Verification items for this drawing (mm, ordinates from the low corner). A direction names the side the tool comes from. Coordinates: 2 decimals unless noted, no trailing zeros. Order: outer loops, then holes, each group sorted by start corner. A loop starts at its lowest first (then second) coordinate and runs counter-clockwise, first axis right, second up. Notation, with made-up numbers: (23.25, 71.5) -> (31.25, 71.5) arc R27 ccw to (31.25, 98.5) -> close; hole circle Ø11 at (-31, 14). An arc over 180 degrees is marked (long way). Write each question's results on one line, items separated by ' | '. Start each with the question number.
(1) Cross-section at D-D on y = 17.75. Enter the section's corners in (x, z).
(2) Cross-section at C-C on y = 2. Enter the section's corners in (x, z) (1 decimal), and give its area (3 significant figures).
(3) Set-up check for the marked faces 1, 2, 3, 4 and 5: record each of +Z, -Z, +X, -X, +Y, -Y from which the full face is reachable in a straight line by a thin tool's end or side.
(4) Thickness scan on probe 1 along Y at (x, z) = (11, 11); probe 2 along X at (y, z) = (1, 9) (3 decimals); probe 3 along Z at (x, y) = (4.5, 2.25). Record the ranges inside material, lowest first. Write a range as [from, to].
(5) Cross-section at A-A on z = 7.5. Enter the section's corners in (x, y) (3 decimals).
(6) Go/stop test with flat-tipped pins: pin 1 (4 mm diameter, centred on y = 10, z = 8, fed in from -X); pin 2 (6 mm diameter, centred on y = 9.5, z = 1.5, fed in from +X) (1 decimal); pin 3 (1.1 mm diameter, centred on y = 2, z = 8, fed in from -X) (3 decimals). Record where each tip stops, or that it passes through.
(7) Cross-section at B-B on x = 9. Enter the section's corners in (y, z).
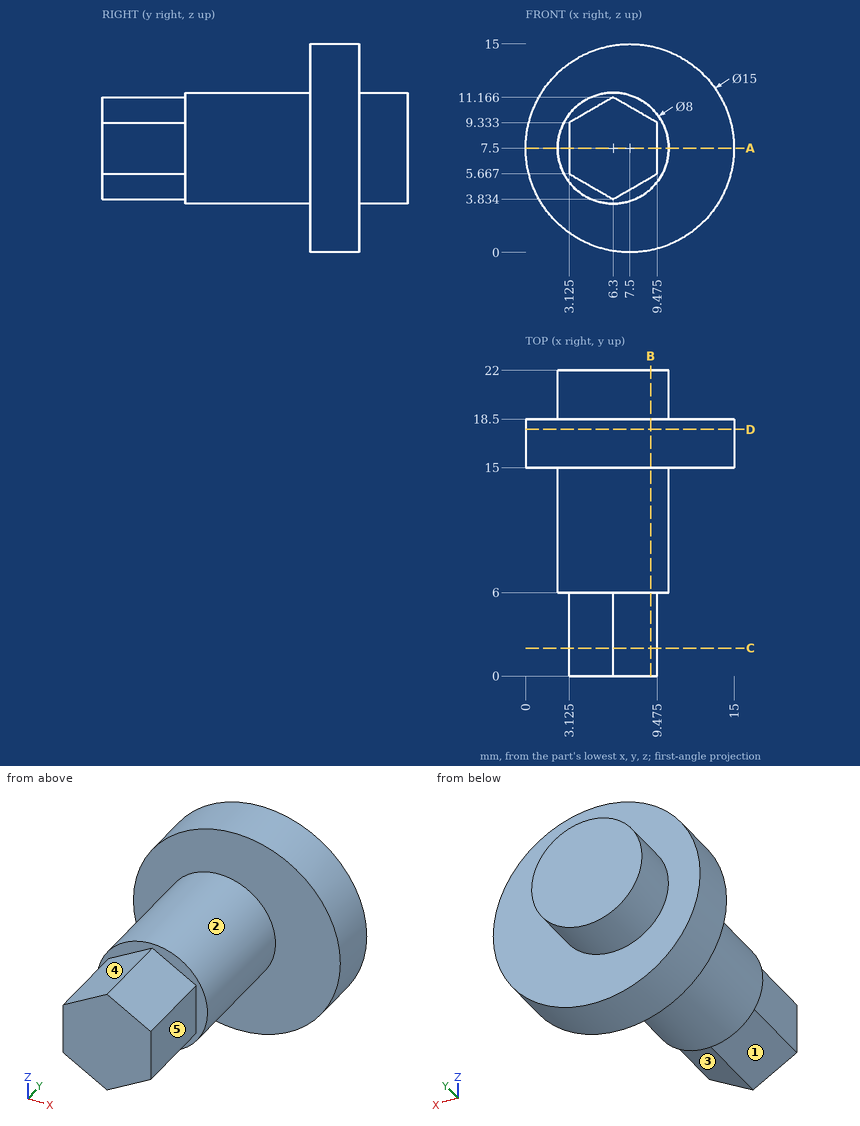
Results are:
1) outline: circle Ø15 at (7.5, 7.5)
2) outline: (3.1, 5.7) -> (6.3, 3.8) -> (9.5, 5.7) -> (9.5, 9.3) -> (6.3, 11.2) -> (3.1, 9.3) -> close | area: 34.9 mm2
3) face 1: -Z, -X, -Y | face 2: -Y | face 3: -Z, +X, -Y | face 4: +Z, -X, -Y | face 5: +Z, -Z, +X, -Y
4) probe 1: y = [15, 18.5] | probe 2: x = [3.125, 9.475] | probe 3: z = [4.87, 10.13]
5) outline: (0, 15) -> (2.3, 15) -> (2.3, 6) -> (3.125, 6) -> (3.125, 0) -> (9.475, 0) -> (9.475, 6) -> (10.3, 6) -> (10.3, 15) -> (15, 15) -> (15, 18.5) -> (10.3, 18.5) -> (10.3, 22) -> (2.3, 22) -> (2.3, 18.5) -> (0, 18.5) -> close
6) pin 1: stops at x = 2.3 | pin 2: stops at x = 8.9 | pin 3: stops at x = 3.125
7) outline: (0, 5.39) -> (6, 5.39) -> (6, 4.55) -> (15, 4.55) -> (15, 0.15) -> (18.5, 0.15) -> (18.5, 4.55) -> (22, 4.55) -> (22, 10.45) -> (18.5, 10.45) -> (18.5, 14.85) -> (15, 14.85) -> (15, 10.45) -> (6, 10.45) -> (6, 9.61) -> (0, 9.61) -> close
